Can you work these out from the model? Positions are in its coordinate system, mm. A direction names the side the tool comes from. Coordinates: 2 decimals unless noted, no trailing zeros. Order: outer loops, then holes, each group sorted by start corner. A loop starts at its lowest first (then second) coordinate and runs counter-clockwise, first axis right, second up. Notation, with made-up numbers: (-39.75, 51.5) -> (11.25, 51.5) arc R29 cw to (11.25, 81.5) -> close; hole circle Ø6 at (59, 82.25). An arc over 180 degrees is marked (long way). Answer in a Markdown table with one row per item. Add a question column.
1. We'd pull the mould along Z, two halves only. Please class faces 1 (the face through (11, 11, 5)), 2 (the face through (0, -7.5, -5)), 3 (the face through (0, -5, -16)): pulls with the +Z half, pulls with the -Z half, needs draft (parallel to the pull), parting line crosses it, or undercut.
2. If I drill on line 1 along Z through (x, y) = (-3.5, 8.75); line 2 along X through (y, z) = (7.25, -14); line 3 along X through (y, z) = (5.25, 8), over which ranges is the centre line in solid material (lowest first)? Write a range as [from, to].
3. On a 3-axis mill with a long thin cutter (end or side, diameter ignored), from which of +Z, -Z, +X, -X, +Y, -Y can I reach the whole of each face in a straight line? I mean faces 4 (the face through (-4.62, -3.66, -13.46)), 5 (the face through (11, -4.9, -11.4)), 6 (the face through (10.14, -10.1, -8.11)). Say none if no direction works.
4. Imagine slicing it at D-D on x = -1. Write out the boundary of the cut face in (y, z), plus the area to 3 significant figures.
5. Imagine slicing it at A-A on x = 27.5. Write out the boundary of the cut face in (y, z).
6. Will these pins go through, and if not, where does the flat tip stop? pin 1 (5 mm diameter, centred on x = 5.66, y = -5.66, fed in from -Z); pin 2 (4 mm diameter, centred on y = 1, z = 7, fed in from +X); pin 3 (6 mm diameter, centred on x = 18, y = 6.5, fed in from -Z); pin 4 (9 mm diameter, centred on x = 0, y = 0, fed in from +Z).
7. Imagine slicing it at C-C on z = 2. Write out the boundary of the cut face in (x, y), plus the area to 3 significant figures.
8. Imagine slicing it at B-B on y = 1. Write out the boundary of the cut face in (x, z), plus the area to 3 significant figures.
from build123d import *

# Parameters (mm, degrees)
SKETCH_R        = 5
SKETCH_R_2      = 1.25
PAD_DEPTH       = 10
SKETCH002_W     = 22
SKETCH002_H     = 3.5
PAD001_DEPTH    = 11
SKETCH003_R     = 4
SKETCH003_R_2   = 2.25
PAD002_DEPTH    = 5
POCKET_DEPTH    = 26.001
POCKET001_DEPTH = 16


with BuildPart() as part:
    # Sketch → Pad (new body)
    with BuildSketch(Plane.XY):
        with BuildLine():
            Line((0, 11), (23, 11))
            ThreePointArc((33.03743, 4.5), (28.97913, 9.233093), (23, 11))
            Line((23, 4.5), (33.03743, 4.5))
            ThreePointArc((23, 4.5), (18.5, 0), (23, -4.5))
            Line((23, -4.5), (33.03743, -4.5))
            ThreePointArc((23, -11), (28.97913, -9.233093), (33.03743, -4.5))
            Line((23, -11), (0, -11))
            Line((-11, -11), (0, -11))
            Line((-11, -11), (-11, 0))
            ThreePointArc((0, 11), (-7.778175, 7.778175), (-11, 0))
        make_face()
        Circle(SKETCH_R, mode=Mode.SUBTRACT)
        with Locations((-5.656854, 5.656854)):
            Circle(SKETCH_R_2, mode=Mode.SUBTRACT)
        with Locations((5.656854, 5.656854)):
            Circle(SKETCH_R_2, mode=Mode.SUBTRACT)
        with Locations((5.656854, -5.656854)):
            Circle(SKETCH_R_2, mode=Mode.SUBTRACT)
        with Locations((-5.656854, -5.656854)):
            Circle(SKETCH_R_2, mode=Mode.SUBTRACT)
    extrude(amount=PAD_DEPTH)

    # Sketch002 (on Face16 of Pad) → Pad001 (join)
    with BuildSketch(Plane(origin=(0, 0, 0), x_dir=(1, 0, 0), z_dir=(0, 0, -1))):
        with Locations((0, 9.25)):
            Rectangle(SKETCH002_W, SKETCH002_H)
    extrude(amount=PAD001_DEPTH)

    # Sketch003 (on Face11 of Pad001) → Pad002 (join)
    with BuildSketch(Plane(origin=(0, 0, -11), x_dir=(1, 0, 0), z_dir=(0, 0, -1))):
        with BuildLine():
            Line((-11, 0), (-11, 11))
            Line((-11, 11), (11, 11))
            Line((11, 11), (11, 0))
            ThreePointArc((-11, 0), (0, -11), (11, 0))
        make_face()
        Circle(SKETCH003_R, mode=Mode.SUBTRACT)
        with Locations((-5.656849, 5.65686)):
            Circle(SKETCH003_R_2, mode=Mode.SUBTRACT)
        with Locations((5.656849, 5.65686)):
            Circle(SKETCH003_R_2, mode=Mode.SUBTRACT)
        with Locations((5.656849, -5.65686)):
            Circle(SKETCH003_R_2, mode=Mode.SUBTRACT)
        with Locations((-5.656871, -5.656837)):
            Circle(SKETCH003_R_2, mode=Mode.SUBTRACT)
    extrude(amount=PAD002_DEPTH)

    # Sketch005 (on Face6 of Pad002) → Pocket (cut, through all)
    with BuildSketch(Plane.XY.offset(10)):
        with BuildLine():
            Line((-11, -11), (-11, -8))
            ThreePointArc((-11, -8), (-10.12132, -10.12132), (-8, -11))
            Line((-11, -11), (-8, -11))
        make_face()
    extrude(amount=-POCKET_DEPTH, mode=Mode.SUBTRACT)

    # Sketch006 (on Face25 of Pocket) → Pocket001 (cut)
    with BuildSketch(Plane(origin=(0, 0, -16), x_dir=(1, 0, 0), z_dir=(0, 0, -1))):
        with BuildLine():
            Line((8, 11), (11, 11))
            Line((11, 11), (11, 8))
            ThreePointArc((11, 8), (10.12132, 10.12132), (8, 11))
        make_face()
    extrude(amount=-POCKET001_DEPTH, mode=Mode.SUBTRACT)


solid = part.part
Answers follow:
| question | item | result |
|---|---|---|
| 1 | face 1 | needs draft |
| 1 | face 2 | undercut |
| 1 | face 3 | pulls with the -Z half |
| 2 | line 1 | z = [-16, -11], [0, 10] |
| 2 | line 2 | x = [-8.27, -7.25], [-4.07, 4.07], [7.25, 8.27] |
| 2 | line 3 | x = [-9.67, -6.84], [-4.47, 4.47], [6.84, 32.67] |
| 3 | face 4 | -Z |
| 3 | face 5 | -Z, +X, +Y, -Y |
| 3 | face 6 | -Z, +X, -Y |
| 4 | outline | (-11, -16) -> (-3.87, -16) -> (-3.87, -11) -> (-7.5, -11) -> (-7.5, 0) -> (-4.9, 0) -> (-4.9, 10) -> (-11, 10) -> close; (3.87, -16) -> (10.95, -16) -> (10.95, -11) -> (3.87, -11) -> close; (4.9, 0) -> (10.95, 0) -> (10.95, 10) -> (4.9, 10) -> close |
| 4 | area | 231 mm² |
| 5 | outline | (-10.04, 0) -> (-4.5, 0) -> (-4.5, 10) -> (-10.04, 10) -> close; (4.5, 0) -> (10.04, 0) -> (10.04, 10) -> (4.5, 10) -> close |
| 6 | pin 1 | stops at z = -16 |
| 6 | pin 2 | stops at x = 19.65 |
| 6 | pin 3 | stops at z = 0 |
| 6 | pin 4 | stops at z = -11 |
| 7 | outline | (-11, -8) arc R3 ccw to (-8, -11) -> (23, -11) arc R11 ccw to (33.04, -4.5) -> (23, -4.5) arc R4.5 cw to (23, 4.5) -> (33.04, 4.5) arc R11 ccw to (23, 11) -> (0, 11) arc R11 ccw to (-11, 0) -> close; hole circle Ø2.5 at (-5.66, -5.66); hole circle Ø2.5 at (-5.66, 5.66); hole circle Ø10 at (0, 0); hole circle Ø2.5 at (5.66, -5.66); hole circle Ø2.5 at (5.66, 5.66) |
| 7 | area | 684 mm² |
| 8 | outline | (-10.95, -16) -> (-3.87, -16) -> (-3.87, -11) -> (-10.95, -11) -> close; (-10.95, 0) -> (-4.9, 0) -> (-4.9, 10) -> (-10.95, 10) -> close; (3.87, -16) -> (10.95, -16) -> (10.95, -11) -> (3.87, -11) -> close; (4.9, 0) -> (18.61, 0) -> (18.61, 10) -> (4.9, 10) -> close |
| 8 | area | 269 mm² |
